from build123d import *

# Parameters (mm, degrees)
F0_R     = 1.5
F1_DEPTH = 3


with BuildPart() as f1:
    # F0 (on Top) → F1 (new body)
    with BuildSketch(Plane.XY):
        with BuildLine():
            Line((0, 6), (0, 0))
            Line((0, 0), (7.4, 0))
            Line((7.4, 0), (7.4, 3))
            Line((7.4, 3), (13.7, 3))
            Line((13.7, 3), (13.7, 0))
            Line((13.7, 0), (20, 0))
            Line((20, 0), (20, 3))
            Line((20, 3), (26.3, 3))
            Line((26.3, 3), (26.3, 0))
            Line((26.3, 0), (29.3, 0))
            Line((29.3, 0), (29.3, 7.75))
            ThreePointArc((29.3, 7.75), (29.51967, 8.28033), (30.05, 8.5))
            Line((30.05, 8.5), (71.6, 8.5))
            Line((71.6, 8.5), (71.6, 14.5))
            Line((71.6, 14.5), (74.6, 14.5))
            Line((74.6, 14.5), (74.6, 20))
            Line((74.6, 20), (71.6, 20))
            Line((71.6, 20), (71.6, 26))
            Line((71.6, 26), (65.35, 26))
            ThreePointArc((65.35, 26), (64.81967, 26.21967), (64.6, 26.75))
            Line((64.6, 26.75), (64.6, 35.25))
            ThreePointArc((64.6, 35.25), (64.81967, 35.78033), (65.35, 36))
            Line((65.35, 36), (71.6, 36))
            Line((71.6, 36), (71.6, 40.5))
            Line((71.6, 40.5), (74.6, 40.5))
            Line((74.6, 40.5), (74.6, 46.3))
            Line((74.6, 46.3), (71.6, 46.3))
            Line((71.6, 46.3), (71.6, 50.8))
            Line((71.6, 50.8), (26.7, 50.8))
            Line((26.7, 50.8), (26.7, 46.95))
            ThreePointArc((26.7, 46.95), (26.48033, 46.41967), (25.95, 46.2))
            Line((25.95, 46.2), (17.45, 46.2))
            ThreePointArc((17.45, 46.2), (16.91967, 46.41967), (16.7, 46.95))
            Line((16.7, 46.95), (16.7, 59.3))
            Line((16.7, 59.3), (13.7, 59.3))
            Line((13.7, 59.3), (13.7, 56.3))
            Line((13.7, 56.3), (7.4, 56.3))
            Line((7.4, 56.3), (7.4, 59.3))
            Line((7.4, 59.3), (0, 59.3))
            Line((0, 59.3), (0, 53.3))
            Line((0, 53.3), (3, 53.3))
            Line((3, 53.3), (3, 47.3))
            Line((3, 47.3), (13.5, 47.3))
            Line((13.5, 47.3), (13.5, 34.3))
            Line((13.5, 34.3), (3, 34.3))
            Line((3, 34.3), (3, 28.1))
            Line((3, 28.1), (0, 28.1))
            Line((0, 28.1), (0, 22))
            Line((0, 22), (3, 22))
            Line((3, 22), (3, 15.8))
            Line((3, 15.8), (16, 15.8))
            Line((16, 15.8), (16, 6))
            Line((16, 6), (0, 6))
        make_face()
        with BuildLine():
            Line((66.75, 15), (31.75, 15))
            ThreePointArc((31.75, 15), (31.21967, 15.21967), (31, 15.75))
            Line((31, 15.75), (31, 23.55))
            ThreePointArc((31, 23.55), (31.21967, 24.08033), (31.75, 24.3))
            Line((31.75, 24.3), (66.75, 24.3))
            ThreePointArc((66.75, 24.3), (67.28033, 24.08033), (67.5, 23.55))
            Line((67.5, 23.55), (67.5, 15.75))
            ThreePointArc((67.5, 15.75), (67.28033, 15.21967), (66.75, 15))
        make_face(mode=Mode.SUBTRACT)
        with BuildLine():
            Line((32.75, 36), (29.25, 36))
            ThreePointArc((29.25, 36), (28.71967, 36.21967), (28.5, 36.75))
            Line((28.5, 36.75), (28.5, 40.25))
            ThreePointArc((28.5, 40.25), (28.71967, 40.78033), (29.25, 41))
            Line((29.25, 41), (32.75, 41))
            ThreePointArc((32.75, 41), (33.28033, 40.78033), (33.5, 40.25))
            Line((33.5, 40.25), (33.5, 36.75))
            ThreePointArc((33.5, 36.75), (33.28033, 36.21967), (32.75, 36))
        make_face(mode=Mode.SUBTRACT)
        with Locations((9.5, 52.3)):
            Circle(F0_R, mode=Mode.SUBTRACT)
        with BuildLine():
            Line((32.75, 43.8), (29.25, 43.8))
            ThreePointArc((29.25, 43.8), (28.71967, 44.01967), (28.5, 44.55))
            Line((28.5, 44.55), (28.5, 46.05))
            ThreePointArc((28.5, 46.05), (28.71967, 46.58033), (29.25, 46.8))
            Line((29.25, 46.8), (32.75, 46.8))
            ThreePointArc((32.75, 46.8), (33.28033, 46.58033), (33.5, 46.05))
            Line((33.5, 46.05), (33.5, 44.55))
            ThreePointArc((33.5, 44.55), (33.28033, 44.01967), (32.75, 43.8))
        make_face(mode=Mode.SUBTRACT)
        with BuildLine():
            Line((62.95, 38.4), (59.45, 38.4))
            ThreePointArc((59.45, 38.4), (58.91967, 38.61967), (58.7, 39.15))
            Line((58.7, 39.15), (58.7, 40.65))
            ThreePointArc((58.7, 40.65), (58.91967, 41.18033), (59.45, 41.4))
            Line((59.45, 41.4), (62.95, 41.4))
            ThreePointArc((62.95, 41.4), (63.48033, 41.18033), (63.7, 40.65))
            Line((63.7, 40.65), (63.7, 39.15))
            ThreePointArc((63.7, 39.15), (63.48033, 38.61967), (62.95, 38.4))
        make_face(mode=Mode.SUBTRACT)
    extrude(amount=-F1_DEPTH)


solid = f1.part
The listing builds one solid part. Answer for the finished solid, in the listing's coordinates (mm). A direction names the side the tool comes from. Coordinates: 2 decimals unless noted, no trailing zeros. Write each loop counter-clockwise with the first axis right and the second up, starting at its lowest first coordinate (ties: lowest second). Pieces come first, ordered by that corner, then holes. Notation, with made-up numbers: M -8.75,59.5 L 32.25,59.5 A25 cw 32.25,87.5 Z; hole C -35,52 d6. An arc over 180 degrees is marked long. Put each result on its own line as item: value. Start each with the question number.
1. A cutting plane is placed at D-D on z = -1.65. Count the separate pieces of the cut face and the enclosed holes in it, then the cut area to 3 significant figures.
2. For a pull along Y with two mould halves and no side action, classify faces 1 (the flat face through (15, 59.3, -1)), 2 (the flat face through (31, 43.8, -1)), 3 (the flat face through (8, 47.3, -1)), 4 (the flat face through (0, 56, -1)) as pulls with the +Y half, pulls with the -Y half, needs draft (parallel to the pull), parting line crosses it, or undercut.
3. A cutting plane is placed at B-B on x = 9.5. Write down the section's boundary in (y, z), then the cut area to 3 significant figures.
4. A cutting plane is placed at A-A on y = 52.3. Write down the section's boundary in (x, z), then the cut area to 3 significant figures.
5. Consider line 1 (Y direction, x = 9.5, z = -1); line 2 (X direction, y = 39.5, z = -1.2); line 3 (Y direction, x = 60, z = -0.35). Determine where each line is inside the solid, lowest interval first. Write a range as from..to.
6. A cutting plane is placed at C-C on x = 53.5. Write down the section's boundary in (y, z).
7. Which of the six approach directions +Z, -Z, +X, -X, +Y, -Y give full straight-line access (tool end or side, diameter ignored) to faces 5 (the flat face through (49, 24.3, -1)), 6 (the flat face through (68, 36, -1)), 7 (the flat face through (11, 56.3, -1)), 8 (the flat face through (71.6, 11, -1))?
8. Flat-ended cylindrical pins translate along their axes: P1, Ø1.5, axis at y = 31, z = -1, coming from the +X side; P2, Ø0.9, axis at x = 43, z = -1.5, coming from the +Y side; P3, Ø1.5, axis at x = 10.5, z = -1, coming from the -Y side. Find the tip coordinate at first contact, or state that the pin passes through.
Resolved:
1. separate pieces: 1
1. enclosed holes: 5
1. area: 2,490 mm2
2. face 1: pulls with the +Y half
2. face 2: undercut
2. face 3: undercut
2. face 4: needs draft
3. outline: M 3,-3 L 6,-3 L 6,0 L 3,0 Z; M 15.8,-3 L 34.3,-3 L 34.3,0 L 15.8,0 Z; M 47.3,-3 L 50.8,-3 L 50.8,0 L 47.3,0 Z; M 53.8,-3 L 56.3,-3 L 56.3,0 L 53.8,0 Z
3. area: 82.5 mm2
4. outline: M 3,-3 L 8,-3 L 8,0 L 3,0 Z; M 11,-3 L 16.7,-3 L 16.7,0 L 11,0 Z
4. area: 32.1 mm2
5. line 1: y = 3..6, 15.8..34.3, 47.3..50.8, 53.8..56.3
5. line 2: x = 13.5..28.5, 33.5..58.7, 63.7..71.6
5. line 3: y = 8.5..15, 24.3..38.4, 41.4..50.8
6. outline: M 8.5,-3 L 15,-3 L 15,0 L 8.5,0 Z; M 24.3,-3 L 50.8,-3 L 50.8,0 L 24.3,0 Z
7. face 5: +Z, -Z
7. face 6: +Z, -Z, +X
7. face 7: +Z, -Z, +Y
7. face 8: +Z, -Z, +X, -Y
8. P1: stops at x = 64.6
8. P2: stops at y = 50.8
8. P3: stops at y = 3
